```python
from build123d import *

# Parameters (mm, degrees)
SKETCH_1_R          = 10
EXTRUDE_1_DEPTH     = 3
SKETCH_2_R          = 5
EXTRUDE_2_DEPTH     = 2
SKETCH_3_R          = 3
SKETCH_3_R_2        = 1
CUT_EXTRUDE_1_DEPTH = 6


with BuildPart() as part:
    # 草图1 → 凸台-拉伸1 (new body)
    with BuildSketch(Plane(origin=(0, 0, 0), x_dir=(1, 0, 0), z_dir=(0, 1, 0))):
        Circle(SKETCH_1_R)
    extrude(amount=EXTRUDE_1_DEPTH)

    # 草图2 → 凸台-拉伸2 (add)
    with BuildSketch(Plane(origin=(0, 3, 0), x_dir=(1, 0, 0), z_dir=(0, 1, 0))):
        Circle(SKETCH_2_R)
    extrude(amount=EXTRUDE_2_DEPTH)

    # 草图3 → 切除-拉伸1 (cut, through all)
    with BuildSketch(Plane.XZ):
        Circle(SKETCH_3_R)
        with Locations((0, 8)):
            Circle(SKETCH_3_R_2)
        with Locations((5.656854249, 5.656854249)):
            Circle(SKETCH_3_R_2)
        with Locations((8, 0)):
            Circle(SKETCH_3_R_2)
        with Locations((5.656854249, -5.656854249)):
            Circle(SKETCH_3_R_2)
        with Locations((0, -8)):
            Circle(SKETCH_3_R_2)
        with Locations((-5.656854249, -5.656854249)):
            Circle(SKETCH_3_R_2)
        with Locations((-8, 0)):
            Circle(SKETCH_3_R_2)
        with Locations((-5.656854249, 5.656854249)):
            Circle(SKETCH_3_R_2)
    extrude(amount=-CUT_EXTRUDE_1_DEPTH, mode=Mode.SUBTRACT)


solid = part.part
```
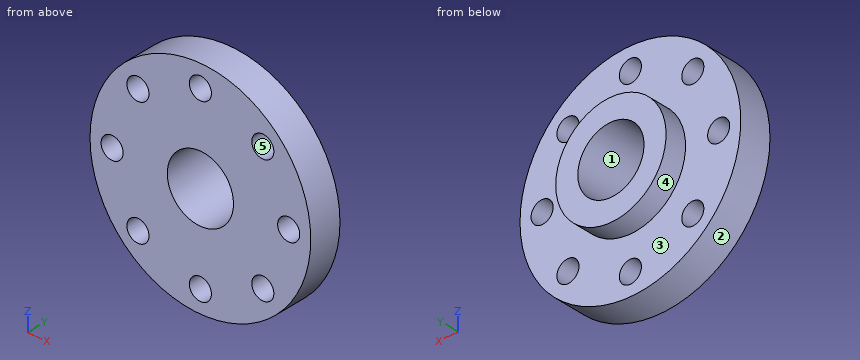
Input: part model. Units: mm. Frame: model coordinates. Face numbers are marked on the shaded views. A direction names the side the tool comes from. Give positions to 0.01 mm unless a question says otherwise; leave off trailing zeros. Write each loop counter-clockwise with the first axis right and the second up, starting at its lowest first coordinate (ties: lowest second). Pieces come first, ordered by that corner, then holes. Notation, with made-up numbers: (-1.75, -21.75) - (9.25, -21.75) arc R25 cw to (9.25, 4.25) - close; hole circle Ø9 at (-29.75, -8). An arc over 180 degrees is marked (long way). Write item = value, one per line. Start each with the question number.
1. Section query B-B, the plane x = -8. Output: boundary loops of the cut face in (y, z).
2. Section query A-A, the plane z = -8. Output: boundary loops of the cut face in (x, y).
3. First-contact query: pin 1 Ø6 at (x, z) = (-2, -1) entering from +Y; pin 2 Ø2.5 at (x, z) = (5.66, 5.66) entering from +Y; pin 3 Ø1.8 at (x, z) = (-5.66, -5.66) entering from -Y. Flat tips, straight axial feed; report the tip coordinate or a pass-through.
4. Access query for the marked faces 4 and 5. Directions: +Z, -Z, +X, -X, +Y, -Y. A direction counts if a zero-diameter tool reaches every point of the face in a straight line with its end or side. Return the directions, or none.
5. Ray query, L1, parallel to Z at x = 0, y = 1.4; L2, parallel to X at y = 0.45, z = 0.75; L3, parallel to Z at x = -5, y = 0.7. Return the intervals inside material, ascending.
6. Section query D-D, the plane z = 0.25. Output: boundary loops of the cut face in (x, y).
7. Mould query, pull axis Z, two halves, no side actions, for the marked faces 1, 2 and 3. Classes: released by +Z, released by -Z, zero draft, split by the parting line, or undercut.
8. Section query C-C, the plane x = 0. Output: boundary loops of the cut face in (y, z), then the cut area to 3 significant figures.
Check sheet entries:
q1.outline = (0, -6) - (3, -6) - (3, -1) - (0, -1) - close; (0, 1) - (3, 1) - (3, 6) - (0, 6) - close
q2.outline = (-6, 0) - (-1, 0) - (-1, 3) - (-6, 3) - close; (1, 0) - (6, 0) - (6, 3) - (1, 3) - close
q3.pin_1 = 5
q3.pin_2 = 3
q3.pin_3 = through
q4.face_4 = +Y
q4.face_5 = +Y, -Y
q5.L1 = -10 to -9, -7 to -3, 3 to 7, 9 to 10
q5.L2 = -9.97 to -8.66, -7.34 to -2.9, 2.9 to 7.34, 8.66 to 9.97
q5.L3 = -8.66 to -6.41, -4.9 to 4.9, 6.41 to 8.66
q6.outline = (-10, 0) - (-8.97, 0) - (-8.97, 3) - (-10, 3) - close; (-7.03, 0) - (-2.99, 0) - (-2.99, 5) - (-4.99, 5) - (-4.99, 3) - (-7.03, 3) - close; (2.99, 0) - (7.03, 0) - (7.03, 3) - (4.99, 3) - (4.99, 5) - (2.99, 5) - close; (8.97, 0) - (10, 0) - (10, 3) - (8.97, 3) - close
q7.face_1 = undercut
q7.face_2 = split by the parting line
q7.face_3 = zero draft
q8.outline = (0, -10) - (3, -10) - (3, -9) - (0, -9) - close; (0, -7) - (3, -7) - (3, -5) - (5, -5) - (5, -3) - (0, -3) - close; (0, 3) - (5, 3) - (5, 5) - (3, 5) - (3, 7) - (0, 7) - close; (0, 9) - (3, 9) - (3, 10) - (0, 10) - close
q8.area = 38.0 mm2
